The figure shows three views and two pictorial views of one solid part (mm, origin at its lowest corner). Answer the questions. A direction names the side the tool comes from. Give positions to 0.01 mm unless a question says otherwise; leave off trailing zeros. Loops run counter-clockwise (first coordinate to the right, second up) from the corner with the lowest first, then second, coordinate; pieces in that order, holes last. Notation, with made-up numbers: (-34, -19) - (-5, -19) arc R38 cw to (-5, 20) - close; hole circle Ø10 at (31.5, 13.25). An arc over 180 degrees is marked (long way). One line per question, with ' | ' between items.
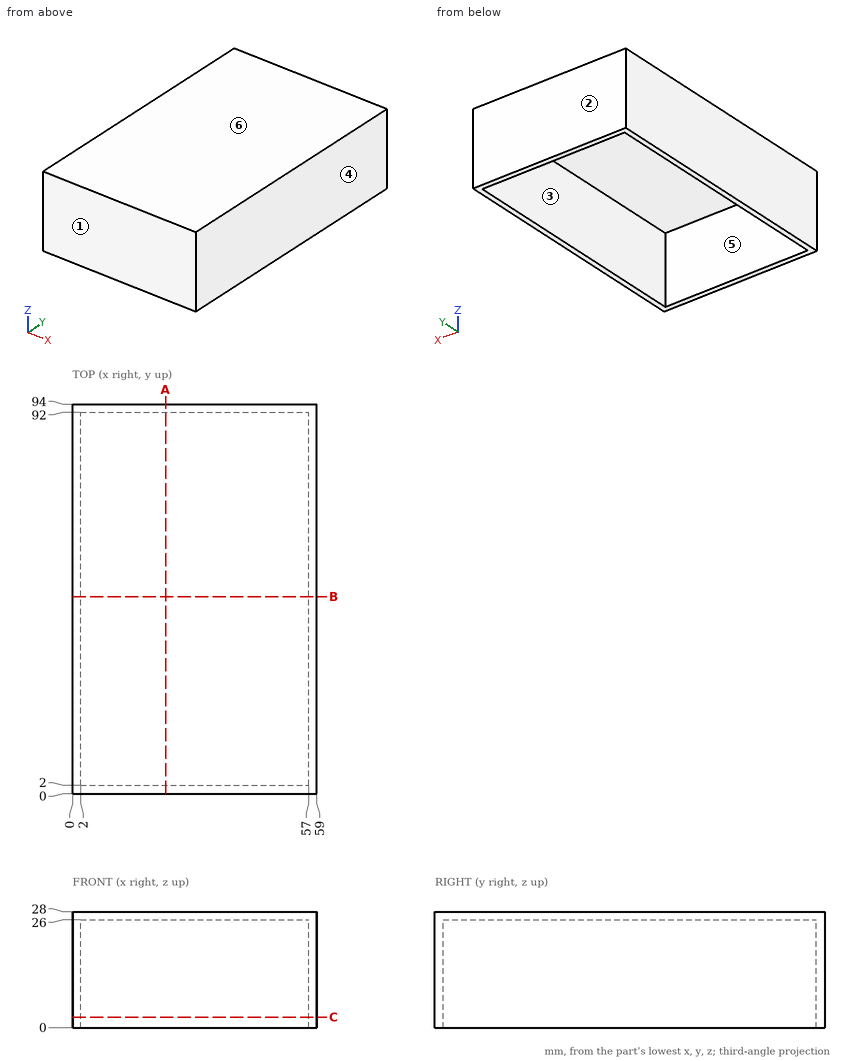
1. Which of the six approach directions +Z, -Z, +X, -X, +Y, -Y give full straight-line access (tool end or side, diameter ignored) to the marked faces 5 and 6?
Evaluation:
face 5: -Z | face 6: +Z, +X, -X, +Y, -Y
2. Consider L1, parallel to Y at x = 29, z = 11.5; L2, parallel to X at y = 31.5, z = 8.5; L3, parallel to Z at x = 15, y = 24. Determine where each line is inside the solid, lowest interval first.
Evaluation:
L1: 0 to 2, 92 to 94 | L2: 0 to 2, 57 to 59 | L3: 26 to 28
3. A flat-ended cylindrical pin translates along its axis: pin 1 (16.5 mm diameter, centred on x = 35, y = 45.5, fed in from -Z). Find the tip coordinate at first contact, or state that the pin passes through.
Evaluation:
pin 1: z = 26
4. Find section A-A on x = 22.5. Write down the section's boundary in (y, z), then the cut area to 3 significant figures.
Evaluation:
outline: (0, 0) - (2, 0) - (2, 26) - (92, 26) - (92, 0) - (94, 0) - (94, 28) - (0, 28) - close | area: 292 mm2
5. Find section B-B on y = 47.5. Write down the section's boundary in (x, z).
Evaluation:
outline: (0, 0) - (2, 0) - (2, 26) - (57, 26) - (57, 0) - (59, 0) - (59, 28) - (0, 28) - close
6. Find section C-C on z = 2.5. Write down the section's boundary in (x, y).
Evaluation:
outline: (0, 0) - (59, 0) - (59, 94) - (0, 94) - close; hole (2, 2) - (57, 2) - (57, 92) - (2, 92) - close
7. Determine the mould class of the marked faces 1, 2, 3 and 4 for opening direction Y: +Y half, -Y half, draft (parallel to the pull), parting line (faces both ways), or undercut.
Evaluation:
face 1: -Y half | face 2: +Y half | face 3: undercut | face 4: draft
